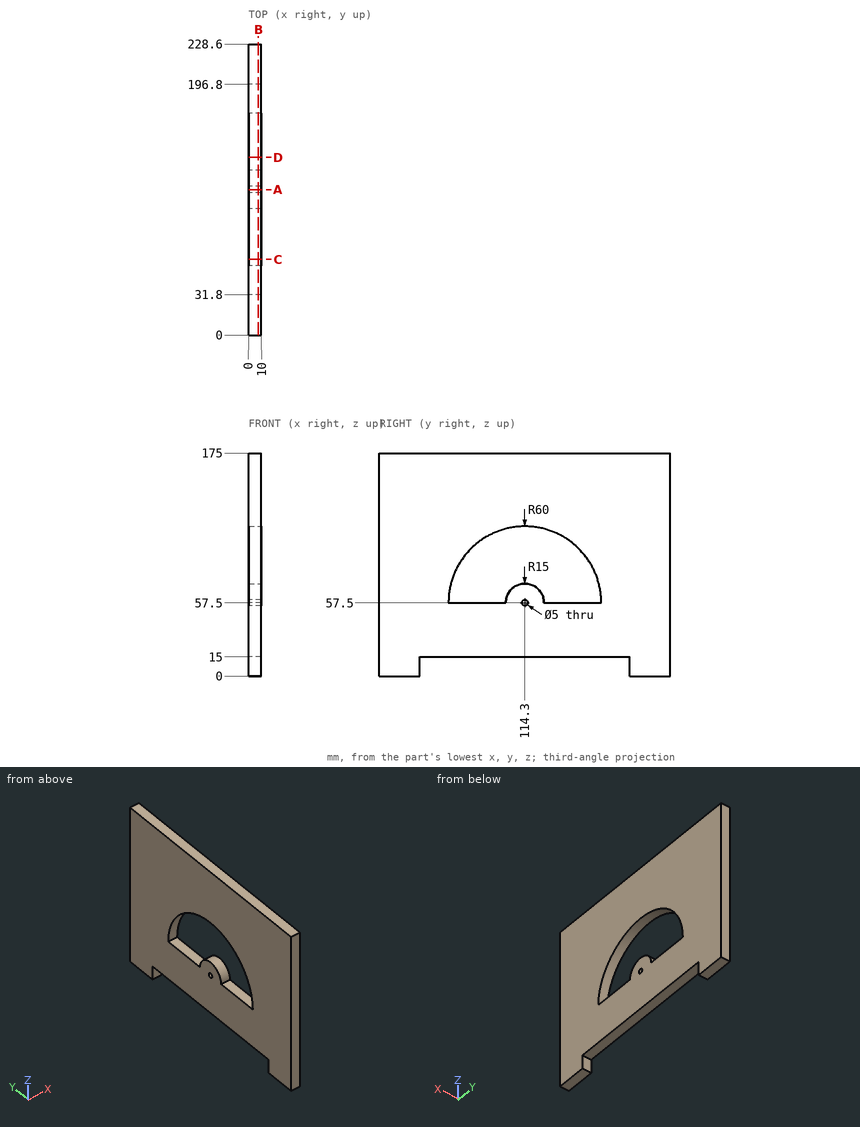
Drawing for the job (mm, zero at the part's lowest x, y, z). Coordinates: 2 decimals unless noted, no trailing zeros. Loops run counter-clockwise (first coordinate to the right, second up) from the corner with the lowest first, then second, coordinate; pieces in that order, holes last. Notation, with made-up numbers: (83.25, 28) - (102.25, 28) arc R36 ccw to (102.25, 66) - close; hole circle Ø6 at (12.5, 73). An arc over 180 degrees is marked (long way). Return JSON: item names as keys, results as strings.
1. Band-saw the part on D-D (y = 139.5). Give the cut face in (x, z).
Result:
{"outline": "(0, 15) - (10, 15) - (10, 57.5) - (0, 57.5) - close; (0, 111.95) - (10, 111.95) - (10, 175) - (0, 175) - close"}
2. Drop a flat-ended pin along its axis: pin 1 (5 mm diameter, centred on x = 5, y = 76.5, fed in from -Z). Give the stop position or say it passes through.
Result:
{"pin 1": "stops at z = 15"}
3. Band-saw the part on A-A (y = 114.3). Give the cut face in (x, z), and give its area (3 significant figures).
Result:
{"outline": "(0, 15) - (10, 15) - (10, 55) - (0, 55) - close; (0, 60) - (10, 60) - (10, 72.5) - (0, 72.5) - close; (0, 117.5) - (10, 117.5) - (10, 175) - (0, 175) - close", "area": "1,100 mm2"}
4. Probe L1, parallel to Z at x = 5.5, y = 114.3; L2, parallel to Y at x = 7.5, z = 61; L3, parallel to Z at x = 9, y = 121.5. List the from-to ranges inside material, lowest first. Write a range as from..to.
Result:
{"L1": "z = 15..55, 60..72.5, 117.5..175", "L2": "y = 0..54.4, 99.71..128.89, 174.2..228.6", "L3": "z = 15..70.66, 117.07..175"}
5. Band-saw the part on B-B (x = 7.75). Give the cut face in (y, z).
Result:
{"outline": "(0, 0) - (31.8, 0) - (31.8, 15) - (196.8, 15) - (196.8, 0) - (228.6, 0) - (228.6, 175) - (0, 175) - close; hole (54.3, 57.5) - (99.3, 57.5) arc R15 cw to (129.3, 57.5) - (174.3, 57.5) arc R60 ccw to start; hole circle Ø5 at (114.3, 57.5)"}
6. Band-saw the part on C-C (y = 59.5). Give the cut face in (x, z), and give its area (3 significant figures).
Result:
{"outline": "(0, 15) - (10, 15) - (10, 57.5) - (0, 57.5) - close; (0, 81.93) - (10, 81.93) - (10, 175) - (0, 175) - close", "area": "1,360 mm2"}
